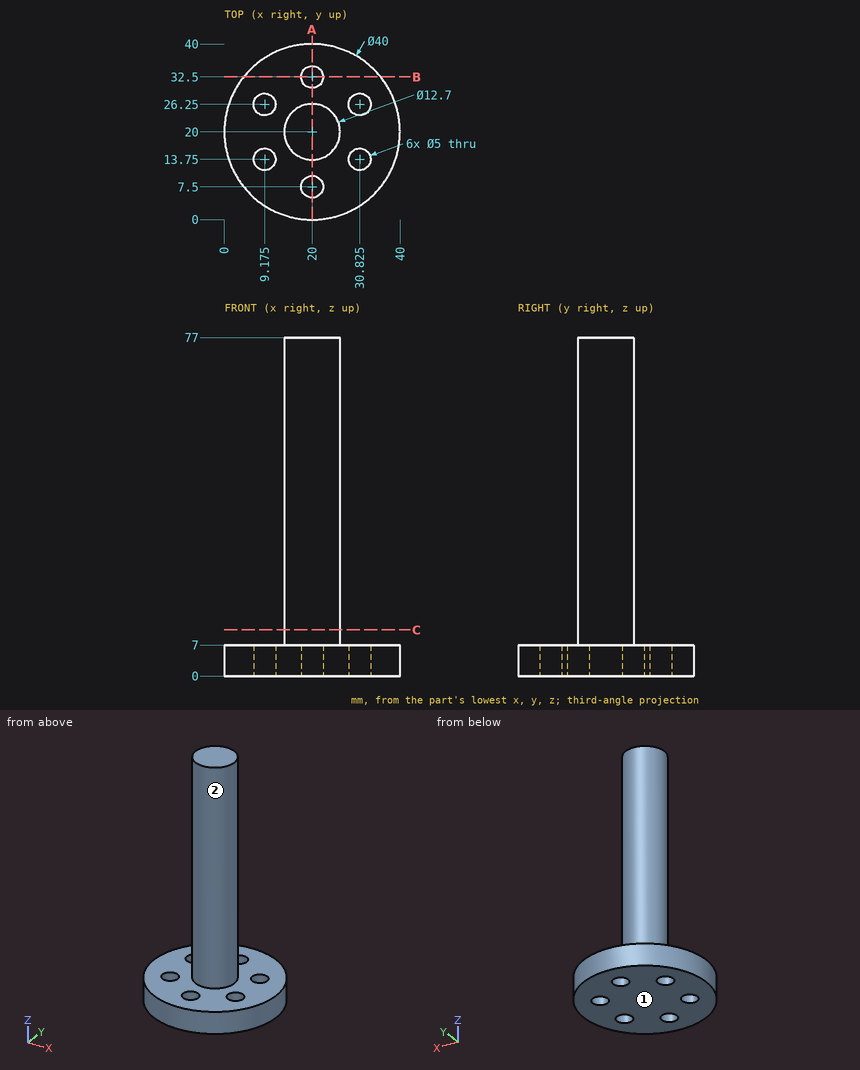
Could you check a few things on this drawing? It's one solid part, dimensions in mm from its lowest x, y, z. A direction names the side the tool comes from. Coordinates: 2 decimals unless noted, no trailing zeros. Order: outer loops, then holes, each group sorted by start corner. A loop starts at its lowest first (then second) coordinate and runs counter-clockwise, first axis right, second up. Notation, with made-up numbers: M 22,25.5 L 53,25.5 A18 ccw 53,37.5 Z; hole C 49.25,22 d4. An arc over 180 degrees is marked long. Use a Markdown table: item, result. Add a question column.
Q1. I want a section at B-B on y = 32.5. List the corners of the cut face in (x, z) for me.
Q2. I want a section at C-C on z = 10.5. List the corners of the cut face in (x, y) for me, then the cut area to 3 significant figures.
Q3. I want a section at A-A on x = 20. List the corners of the cut face in (y, z) for me.
Q4. Which directions (+Z, -Z, +X, -X, +Y, -Y) give clear straight access to the entire face, cutting with the end or side of a thin tool? Please do the marked faces 1 and 2.
Q5. If I drill on L1, parallel to Y at x = 7.5, z = 6.5 (1 decimal); L2, parallel to X at y = 13, z = 1 (1 decimal); L3, parallel to Z at x = 6, y = 17, over which ranges is the centre line in solid material (lowest first)?
Q6. I'm going to push flat-ended pins straight in: pin 1 (10 mm diameter, centred on x = 16.5, z = 33.5, fed in from +Y); pin 2 (8 mm diameter, centred on x = 30.83, y = 13.75, fed in from +Z); pin 3 (1 mm diameter, centred on y = 23.5, z = 64, fed in from +X). Where does each tip first touch, or does it pass through?
Checked values:
| question | item | result |
|---|---|---|
| 1 | outline | M 4.39,0 L 17.5,0 L 17.5,7 L 4.39,7 Z; M 22.5,0 L 35.61,0 L 35.61,7 L 22.5,7 Z |
| 2 | outline | C 20,20 d12.7 |
| 2 | area | 127 mm² |
| 3 | outline | M 0,0 L 5,0 L 5,7 L 0,7 Z; M 10,0 L 30,0 L 30,7 L 26.35,7 L 26.35,77 L 13.65,77 L 13.65,7 L 10,7 Z; M 35,0 L 40,0 L 40,7 L 35,7 Z |
| 4 | face 1 | -Z, +X, -X, +Y, -Y |
| 4 | face 2 | +Z |
| 5 | L1 | 4.4 to 11.9, 15.6 to 24.4, 28.1 to 35.6 |
| 5 | L2 | 1.3 to 6.8, 11.6 to 28.4, 33.2 to 38.7 |
| 5 | L3 | 0 to 7 |
| 6 | pin 1 | y = 26.35 |
| 6 | pin 2 | z = 7 |
| 6 | pin 3 | x = 25.6 |
